Design review of the part built by this model. Coordinates are the model's own, in mm. A direction names the side the tool comes from. Coordinates: 2 decimals unless noted, no trailing zeros. Write each loop counter-clockwise with the first axis right and the second up, starting at its lowest first coordinate (ties: lowest second). Pieces come first, ordered by that corner, then holes.
Q1. To check wall thickness, follow probe 1 along Y at (x, z) = (16.5, -5.5); probe 2 along Y at (x, z) = (157.5, -6.6). State the ranges of each line that lie inside material, in increasing order.
Q2. Add section C-C, the plane x = 172.5. Give the boundary of the cut face in (y, z).
Q3. Machinability: for faces 5 (the face through (89, 6, 0)), 6 (the face through (0, 0, 7)), which of the approach directions +Z, -Z, +X, -X, +Y, -Y give a long, thin tool a straight path to every point of the face, cutting with its end or side? Answer none if there is none.
Q4. Add section A-A, the plane x = 149. Give the boundary of the cut face in (y, z).
Q5. Add section D-D, the plane y = 0. Give the number of separate pieces and of enclosed holes in the cut face, plus the area to 3 significant figures.
Q6. Add section B-B, the plane z = -2.25. Give the boundary of the cut face in (x, y).
Q7. Clearance check with a flat-ended pin moving along its axis: pin 1 Ø3.5 at (x, y) = (172.5, 0) entering from +Z. State where the tip first meets the part, or that it passes through.
Q8. The part is to be moulded in two halves that separate along Z. For faces 1 (the face through (89, -3, 7.5)), 2 (the face through (89, 7.5, 0)), 3 (the face through (89, 3, 6)), 4 (the face through (89, -3, -7.5)), say which applies: +Z half, -Z half, draft (parallel to the pull), parting line (faces both ways), or undercut.
from build123d import *

# Parameters (mm, degrees)
SKETCH_1_W          = 15
SKETCH_1_H          = 15
SKETCH_1_W_2        = 12
SKETCH_1_H_2        = 12
EXTRUDE_1_DEPTH     = 180
SKETCH_2_R          = 2.1
CUT_EXTRUDE_1_DEPTH = 181.779561898


with BuildPart() as part:
    # ｽｹｯﾁ1 → 押し出し-薄板1 (new body)
    with BuildSketch(Plane(origin=(0, 0, 0), x_dir=(0, 0, -1), z_dir=(1, 0, 0))):
        Rectangle(SKETCH_1_W, SKETCH_1_H)
        Rectangle(SKETCH_1_W_2, SKETCH_1_H_2, mode=Mode.SUBTRACT)
    extrude(amount=EXTRUDE_1_DEPTH)

    # ｽｹｯﾁ2 → ｶｯﾄ - 押し出し1 (cut, through all)
    with BuildSketch(Plane.XY.offset(7.5)):
        with Locations((22.5, 0)):
            Circle(SKETCH_2_R)
        with Locations((7.5, 0)):
            Circle(SKETCH_2_R)
        with Locations(Location((172.5, 0, 0), (0, 0, 90))):
            Circle(SKETCH_2_R)
        with Locations(Location((157.5, 0, 0), (0, 0, 90))):
            Circle(SKETCH_2_R)
        with Locations((90, 0)):
            Circle(SKETCH_2_R)
    extrude(amount=-CUT_EXTRUDE_1_DEPTH, mode=Mode.SUBTRACT)


solid = part.part
Here are the results:
1. probe 1: y = -7.5 to -6, 6 to 7.5
1. probe 2: y = -7.5 to -2.1, 2.1 to 7.5
2. outline: (-7.5, -7.5) - (-2.1, -7.5) - (-2.1, -6) - (-6, -6) - (-6, 6) - (-2.1, 6) - (-2.1, 7.5) - (-7.5, 7.5) - close; (2.1, -7.5) - (7.5, -7.5) - (7.5, 7.5) - (2.1, 7.5) - (2.1, 6) - (6, 6) - (6, -6) - (2.1, -6) - close
3. face 5: +X, -X
3. face 6: +Z, -Z, -X, +Y, -Y
4. outline: (-7.5, -7.5) - (7.5, -7.5) - (7.5, 7.5) - (-7.5, 7.5) - close; hole (-6, -6) - (6, -6) - (6, 6) - (-6, 6) - close
5. separate pieces: 12
5. enclosed holes: 0
5. area: 477 mm2
6. outline: (0, -7.5) - (180, -7.5) - (180, -6) - (0, -6) - close; (0, 6) - (180, 6) - (180, 7.5) - (0, 7.5) - close
7. pin 1: passes through
8. face 1: +Z half
8. face 2: draft
8. face 3: undercut
8. face 4: -Z half
